Verification items for the finished model (mm, model axes). Face numbers are marked on the shaded views. Round coordinates to 2 decimals unless told otherwise and drop trailing zeros. Order: outer loops, then holes, each group sorted by start corner. A loop starts at its lowest first (then second) coordinate and runs counter-clockwise, first axis right, second up. Notation, with made-up numbers: M -7.75,14.25 L -0.75,14.25 A21 cw -0.75,25.25 Z; hole C 26,49 d10. An arc over 180 degrees is marked long. Answer as a JSON object with one key per item and string values. Group by question number.
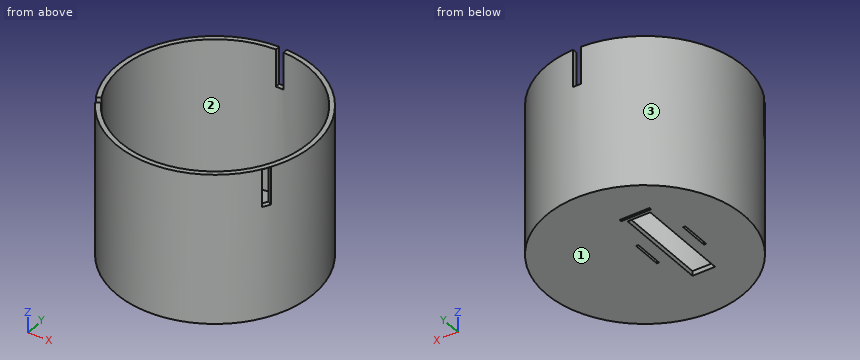
```python
from build123d import *

# Parameters (mm, degrees)
F0_R           = 33.3375
F1_DEPTH       = 50.8
F2_T           = -1.5875
F6_W           = 2.5429241359
F6_H           = 13.1887868047
F7_DEPTH       = 12.7
F10_W          = 2.6744855568
F10_H          = 12.775093317
F11_DEPTH      = 2.794
F11_DEPTH_BACK = 2.413
F13_W          = 2.5820170995
F13_H          = 12.7615630627
F14_DEPTH      = 5.0546
F14_DEPTH_BACK = 4.7244
F15_W          = 7.62
F15_H          = 31.75
F15_W_2        = 0.7620003967
F15_H_2        = 10.16
F15_W_3        = 0.762
F15_W_4        = 10.16
F15_H_3        = 0.762
F16_DEPTH      = 9.906


with BuildPart() as f1:
    # F0 (on Top) → F1 (new body)
    with BuildSketch(Plane.XY):
        Circle(F0_R)
    extrude(amount=F1_DEPTH)

    # F2
    f2_openings = [f1.faces().sort_by_distance(p)[0] for p in [
        (0, 0, 50.8),
    ]]
    offset(amount=F2_T, openings=f2_openings)

    # F6 (on offset) → F7 (cut)
    with BuildSketch(Plane(origin=(-28.8711218987, -16.66875, 0), x_dir=(0.5, -0.8660254038, 0), z_dir=(-0.8660254038, -0.5, 0))):
        with Locations((0, 44.4019660354)):
            Rectangle(F6_W, F6_H)
    extrude(amount=-F7_DEPTH, mode=Mode.SUBTRACT)

    # F10 (on offset) → F11 (cut, two sides)
    with BuildSketch(Plane(origin=(28.8161292855, -16.637, 0), x_dir=(0.5, 0.8660254038, 0), z_dir=(0.8660254038, -0.5, 0))) as f11_sk:
        with Locations((0, 44.3391613662)):
            Rectangle(F10_W, F10_H)
    extrude(amount=-F11_DEPTH, mode=Mode.SUBTRACT)
    extrude(f11_sk.sketch, amount=F11_DEPTH_BACK, mode=Mode.SUBTRACT)

    # F13 (on offset) → F14 (cut, two sides)
    with BuildSketch(Plane.XZ.offset(-33.81375)) as f14_sk:
        with Locations((0, 44.5175170898)):
            Rectangle(F13_W, F13_H)
    extrude(amount=-F14_DEPTH, mode=Mode.SUBTRACT)
    extrude(f14_sk.sketch, amount=F14_DEPTH_BACK, mode=Mode.SUBTRACT)

    # F15 (on Top) → F16 (cut)
    with BuildSketch(Plane.XY):
        with Locations((-8.89, 0)):
            Rectangle(F15_W, F15_H)
        with Locations((-0.6896582572, -0.2738600914)):
            Rectangle(F15_W_2, F15_H_2)
        with Locations((-16.5646602053, -0.2738598244)):
            Rectangle(F15_W_3, F15_H_2)
        with Locations((-8.6557281865, 17.3283369606)):
            Rectangle(F15_W_4, F15_H_3)
    extrude(amount=F16_DEPTH, mode=Mode.SUBTRACT)


solid = f1.part
```
Q1. Cross-section at D-D, the plane y = -12. Record the cut outline in (x, z).
Q2. Gauge pin test, flat ends, axial feed: pin 1 Ø6 at (y, z) = (-21.5, 31.5) entering from -X; pin 2 Ø0.8 at (y, z) = (17.5, 0.5) entering from -X; pin 3 Ø12 at (y, z) = (-6.5, 28) entering from +X. Record the tip position at first contact, or that the pin passes through.
Q3. Cross-section at C-C, the plane x = 22. Record the cut outline in (y, z).
Q4. Thickness scan on line 1 (Y direction, x = 0, z = 34); line 2 (Z direction, x = -4, y = 4). Record the ranges inside material, lowest first. Write a range as from..to.
Q5. Release check for a two-part mould opening along X. For the marked faces 1, 2 and 3 record: released by +X, released by -X, zero draft, split by the parting line, or undercut.
Q6. Cross-section at A-A, the plane y = 0. Record the cut outline in (x, z).
Conclusion:
{
 "1": {"outline": "M -31.1,0 L -12.7,0 L -12.7,1.59 L -29.39,1.59 L -29.39,50.8 L -31.1,50.8 Z; M -5.08,0 L 31.1,0 L 31.1,50.8 L 29.39,50.8 L 29.39,1.59 L -5.08,1.59 Z"},
 "2": {"pin 1": "x = -27.73", "pin 2": "x = -28.62", "pin 3": "x = 33.33"},
 "3": {"outline": "M -25.05,0 L 25.05,0 L 25.05,50.8 L 22.89,50.8 L 22.89,1.59 L -22.89,1.59 L -22.89,50.8 L -25.05,50.8 Z"},
 "4": {"line 1": "-33.34..-31.75, 31.75..33.34", "line 2": "0..1.59"},
 "5": {"face 1": "zero draft", "face 2": "undercut", "face 3": "split by the parting line"},
 "6": {"outline": "M -33.34,0 L -16.95,0 L -16.95,1.59 L -31.75,1.59 L -31.75,50.8 L -33.34,50.8 Z; M -16.18,0 L -12.7,0 L -12.7,1.59 L -16.18,1.59 Z; M -5.08,0 L -1.07,0 L -1.07,1.59 L -5.08,1.59 Z; M -0.31,0 L 33.34,0 L 33.34,50.8 L 31.75,50.8 L 31.75,1.59 L -0.31,1.59 Z"}
}
